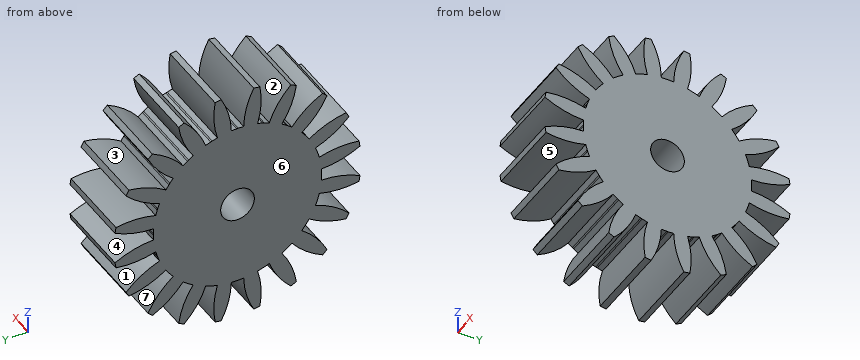
from build123d import *

# Parameters (mm, degrees)
SKETCH1_R                = 110
BOSS_EXTRUDE1_DEPTH      = 35
SKETCH6_R                = 15
CUT_EXTRUDE4_DEPTH       = 171.587221092
CUT_EXTRUDE5_DEPTH       = 171.587221092
FILLET1_R                = 20
CIRPATTERN3_COUNT        = 20
FILLET1_OF_CIRPATTERN3_R = 20


with BuildPart() as part:
    # Sketch1 → Boss-Extrude1 (new, symmetric)
    with BuildSketch(Plane(origin=(0, 0, 0), x_dir=(0, 0, -1), z_dir=(1, 0, 0))):
        Circle(SKETCH1_R)
    extrude(amount=BOSS_EXTRUDE1_DEPTH, both=True)

    # Sketch6 → Cut-Extrude4 (cut, through all)
    with BuildSketch(Plane(origin=(35, 0, 0), x_dir=(0, 0, -1), z_dir=(1, 0, 0))):
        Circle(SKETCH6_R)
    extrude(amount=-CUT_EXTRUDE4_DEPTH, mode=Mode.SUBTRACT)

    # Sketch7 → Cut-Extrude5 (cut, through all)
    with BuildSketch(Plane(origin=(35, 0, 0), x_dir=(0, 0, -1), z_dir=(1, 0, 0))):
        with BuildLine():
            Line((0, 74.98517078), (-5.5, 74.798061472))
            ThreePointArc((-5.5, 74.798061472), (-7.995035607, 92.446069838), (-14.5, 109.040130227))
            Line((-14.5, 109.040130227), (0, 147))
            Line((0, 147), (14.5, 109.040130227))
            ThreePointArc((14.5, 109.040130227), (7.995035607, 92.446069838), (5.5, 74.798061472))
            Line((5.5, 74.798061472), (0, 74.98517078))
        make_face()
    cut_extrude5 = extrude(amount=-CUT_EXTRUDE5_DEPTH, mode=Mode.SUBTRACT)

    # Fillet1
    # the kernel refuses this fillet: 20 mm, written as the material it takes off along each edge
    with BuildSketch(Plane(origin=(36.700993707, 74.98517078, 0), x_dir=(0, -0.034000204734020274, -0.9994218258963753), z_dir=(-1, 0, 0))) as fillet1_piece_1:
        with BuildLine():
            CenterArc((FILLET1_R * 0.0340198741443, FILLET1_R), FILLET1_R, 266.103112477, 3.896887523)
            Line((-FILLET1_R * 0.033941219248, FILLET1_R * 0.00231202784391), (0, 0))
            Line((0, 0), (FILLET1_R * 0.0340198741443, 0))
        make_face()
    extrude(amount=73.401987414, mode=Mode.SUBTRACT)

    # CirPattern3: Cut-Extrude5 ×20 about axis
    cirpattern3_axis = Axis((0, 0, 0), (1, 0, 0))
    for i in range(1, CIRPATTERN3_COUNT):
        add(cut_extrude5.rotate(cirpattern3_axis, i * 360 / CIRPATTERN3_COUNT), mode=Mode.SUBTRACT)

    # Fillet1 of CirPattern3
    # the kernel refuses this fillet: 20 mm, written as the material it takes off along each edge
    with BuildSketch(Plane(origin=(36.700993707, 71.315135296, 23.171692097), x_dir=(0, -0.3411744450188669, 0.9399999989713128), z_dir=(-1, 0, 0)), Plane(origin=(36.700993707, 60.664277487, 44.075177525), x_dir=(0, -0.6149521535231338, 0.7885644227818424), z_dir=(-1, 0, 0)), Plane(origin=(36.700993707, 44.075177525, 60.664277487), x_dir=(0, -0.8285340606169823, 0.5599386666390654), z_dir=(-1, 0, 0)), Plane(origin=(36.700993707, 23.171692097, 71.315135296), x_dir=(0, -0.9610132811213845, 0.2765022124835726), z_dir=(-1, 0, 0)), Plane(origin=(36.700993707, 0, 74.98517078), x_dir=(0, -0.9994218258963753, -0.03400020473402028), z_dir=(-1, 0, 0)), Plane(origin=(36.700993707, -23.171692097, 71.315135296), x_dir=(0, -0.9399999989713128, -0.3411744450188669), z_dir=(-1, 0, 0)), Plane(origin=(36.700993707, -44.075177525, 60.664277487), x_dir=(0, -0.7885644227818294, -0.6149521535231504), z_dir=(-1, 0, 0)), Plane(origin=(36.700993707, -60.664277487, 44.075177525), x_dir=(0, -0.5599386666390632, -0.8285340606169839), z_dir=(-1, 0, 0)), Plane(origin=(36.700993707, -71.315135296, 23.171692097), x_dir=(0, -0.2765022124835726, -0.9610132811213845), z_dir=(-1, 0, 0)), Plane(origin=(36.700993707, -74.98517078, 0), x_dir=(0, 0.0340002047340203, -0.9994218258963753), z_dir=(-1, 0, 0)), Plane(origin=(36.700993707, -71.315135296, -23.171692097), x_dir=(0, 0.34117444501886857, -0.9399999989713121), z_dir=(-1, 0, 0)), Plane(origin=(36.700993707, -60.664277487, -44.075177525), x_dir=(0, 0.6149521535231454, -0.7885644227818334), z_dir=(-1, 0, 0)), Plane(origin=(36.700993707, -44.075177525, -60.664277487), x_dir=(0, 0.8285340606169823, -0.5599386666390654), z_dir=(-1, 0, 0)), Plane(origin=(36.700993707, -23.171692097, -71.315135296), x_dir=(0, 0.9610132811213842, -0.276502212483574), z_dir=(-1, 0, 0)), Plane(origin=(36.700993707, 0, -74.98517078), x_dir=(0, 0.9994218258963753, 0.034000204734020295), z_dir=(-1, 0, 0)), Plane(origin=(36.700993707, 23.171692097, -71.315135296), x_dir=(0, 0.939999998971314, 0.34117444501886357), z_dir=(-1, 0, 0)), Plane(origin=(36.700993707, 44.075177525, -60.664277487), x_dir=(0, 0.7885644227818333, 0.6149521535231453), z_dir=(-1, 0, 0)), Plane(origin=(36.700993707, 60.664277487, -44.075177525), x_dir=(0, 0.559938666639056, 0.8285340606169888), z_dir=(-1, 0, 0)), Plane(origin=(36.700993707, 71.315135296, -23.171692097), x_dir=(0, 0.2765022124835726, 0.9610132811213845), z_dir=(-1, 0, 0))) as fillet1_of_cirpattern3_piece_1:
        with BuildLine():
            CenterArc((FILLET1_OF_CIRPATTERN3_R * 0.0340198741442, -FILLET1_OF_CIRPATTERN3_R), FILLET1_OF_CIRPATTERN3_R, 90, 3.896887523)
            Line((-FILLET1_OF_CIRPATTERN3_R * 0.033941219248, -FILLET1_OF_CIRPATTERN3_R * 0.00231202784391), (0, 0))
            Line((0, 0), (FILLET1_OF_CIRPATTERN3_R * 0.0340198741443, 0))
        make_face()
    extrude(amount=73.401987414, mode=Mode.SUBTRACT)


solid = part.part
Work out the finished part from the listing and answer in its coordinate system (mm). Face numbers are marked on the shaded views. A direction names the side the tool comes from. Round coordinates to 2 decimals unless told otherwise and drop trailing zeros. Loops run counter-clockwise (first coordinate to the right, second up) from the corner with the lowest first, then second, coordinate; pieces in that order, holes last. Notation, with made-up numbers: (81, 73.25) - (105, 73.25) arc R15 cw to (105, 102.25) - close; hole circle Ø5 at (42.5, -40). An arc over 180 degrees is marked (long way). One line per item, written item: value.
Q1. Find section D-D on y = -31. Give the vertices of the cut face in (x, z).
Check values:
outline: (-35, -76) - (35, -76) - (35, 76) - (-35, 76) - close
Q2. Find section B-B on z = 91. Give the vertices of the cut face in (x, y).
Check values:
outline: (-35, -51.34) - (35, -51.34) - (35, -40.1) - (-35, -40.1) - close; (-35, -21) - (35, -21) - (35, -7.63) - (-35, -7.63) - close; (-35, 7.63) - (35, 7.63) - (35, 21) - (-35, 21) - close; (-35, 40.1) - (35, 40.1) - (35, 51.34) - (-35, 51.34) - close
Q3. Each of these flat-tipped pins is pushed along its axis until it touches: pin 1 Ø2 at (x, y) = (-6.5, 38) entering from -Z; pin 2 Ø3 at (x, z) = (3, -73.5) entering from -Y; pin 3 Ø10 at (x, y) = (1, 70) entering from -Z. Where does it stop, or does it pass through?
Check values:
pin 1: z = -89.55
pin 2: y = -79.29
pin 3: z = -79.29
Q4. Find section C-C on y = 85. Give the vertices of the cut face in (x, z), and give its area (3 significant figures).
Check values:
outline: (-35, -49.78) - (35, -49.78) - (35, -35.88) - (-35, -35.88) - close; (-35, -20.46) - (35, -20.46) - (35, -6.43) - (-35, -6.43) - close; (-35, 6.43) - (35, 6.43) - (35, 20.46) - (-35, 20.46) - close; (-35, 35.88) - (35, 35.88) - (35, 49.78) - (-35, 49.78) - close
area: 3,910 mm2
Q5. The mould has two halves that part along Y. Classify the marked faces 4, 5, 6 and 7: +Y half, -Y half, draft (parallel to the pull), parting line (faces both ways), or undercut.
Check values:
face 4: +Y half
face 5: undercut
face 6: draft
face 7: undercut
Q6. For the marked faces 1, 2 and 3, determine the directions among +Z, -Z, +X, -X, +Y, -Y from which every point of the face is accessible in a straight line to the end or side of a thin tool.
Check values:
face 1: +X, -X, +Y
face 2: +Z, +X, -X
face 3: +X, -X
Q7. Straight lines are drawn through the part: probe 1 along Y at (x, z) = (18, -82); probe 2 along Z at (x, y) = (8, -98.5); probe 3 along Z at (x, y) = (-25, -64.5). For each, find the intervals that lie inside material, in ascending order.
Check values:
probe 1: -48.8 to -34.08, -20.02 to -6.01, 6.01 to 20.02, 34.08 to 48.8
probe 2: -48.97 to -46.75, -21 to -9.86, 9.86 to 21, 46.75 to 48.97
probe 3: -72.93 to -54.68, -40.03 to 40.03, 54.68 to 72.93
Q8. Find section A-A on z = 11. Give the vertices of the cut face in (x, y), and give its area (3 significant figures).
Check values:
outline: (-35, -101.53) - (35, -101.53) - (35, -10.2) - (-35, -10.2) - close; (-35, 10.2) - (35, 10.2) - (35, 101.53) - (-35, 101.53) - close
area: 12,800 mm2
